Geometry: final body of the model. Coordinates: model frame, mm. A direction names the side the tool comes from. Coordinates: 2 decimals unless noted, no trailing zeros. Order: outer loops, then holes, each group sorted by start corner. A loop starts at its lowest first (then second) coordinate and runs counter-clockwise, first axis right, second up. Notation, with made-up numbers: M 41,88.5 L 87,88.5 A20 ccw 87,100.5 Z; hole C 82.25,89 d5. An arc over 180 degrees is marked long. Write item = value, one per line. Start each with the question number.
```python
from build123d import *

# Parameters (mm, degrees)
BOSS_EXTRUDE1_DEPTH    = 10
LPATTERN1_COUNT        = 2
LPATTERN1_PITCH        = 80
SKETCH2_W              = 69.30058394
SKETCH2_H              = 90
BOSS_EXTRUDE2_DEPTH    = 7
SKETCH3_R              = 2.5
CUT_EXTRUDE1_DEPTH     = 10
BOSS_EXTRUDE3_DEPTH    = 77
CUT_EXTRUDE2_START     = -2.5
CUT_EXTRUDE2_OUTLINE_W = 20.397762745
CUT_EXTRUDE2_OUTLINE_H = 50
CUT_EXTRUDE2_OUTLINE_R = 2.05
CUT_EXTRUDE2_DEPTH     = 2.5


# Read off the part's stored shape, not the designer's step: Cut-Extrude2
with BuildPart() as part:
    # Sketch1 → Boss-Extrude1 (new body)
    with BuildSketch(Plane.XY):
        Polygon((0, 0), (11.349310372, 59.718827606), (30.34970803, 100), (99.65029197, 100), (118.650689628, 59.718827606), (130, 0), (120, 0), (109.631710362, 54.556803995), (91.49827561, 93), (38.50172439, 93), (20.368289638, 54.556803995), (10, 0), align=None)
    extrude(amount=BOSS_EXTRUDE1_DEPTH)


with BuildPart() as lpattern1_1:
    # LPattern1: pattern copy
    add(part.part.moved(Location(Vector(0, 0, -1) * (1 * LPATTERN1_PITCH))))


with BuildPart() as part_1:
    add(part.part)

    add(lpattern1_1.part)  # Boss-Extrude2 merges LPattern1_1
    # Sketch2 → Boss-Extrude2 (add)
    with BuildSketch(Plane(origin=(0, 100, 0), x_dir=(1, 0, 0), z_dir=(0, 1, 0))):
        with Locations((65, 35)):
            Rectangle(SKETCH2_W, SKETCH2_H)
    extrude(amount=-BOSS_EXTRUDE2_DEPTH)

    # Sketch3 → Cut-Extrude1 (cut)
    with BuildSketch(Plane.XZ.offset(-93)):
        with Locations(Location((65, -35, 0), (0, 0, 270))):
            Circle(SKETCH3_R)
    extrude(amount=-CUT_EXTRUDE1_DEPTH, mode=Mode.SUBTRACT)

    # Sketch4 → Boss-Extrude3 (add)
    with BuildSketch(Plane.XY.offset(-70)):
        Polygon((130, 0), (129.524885584, 2.5), (119.524885584, 2.5), (120, 0), align=None)
        Polygon((0, 0), (10, 0), (10.475114416, 2.5), (0.475114416, 2.5), align=None)
    extrude(amount=BOSS_EXTRUDE3_DEPTH)

    # Cut-Extrude2 outline → Cut-Extrude2 (cut)
    with BuildSketch(Plane(origin=(0, 2.5, 0), x_dir=(1, 0, 0), z_dir=(0, 1, 0)).offset(CUT_EXTRUDE2_START)):
        with Locations((129.723766957, 35)):
            Rectangle(CUT_EXTRUDE2_OUTLINE_W, CUT_EXTRUDE2_OUTLINE_H)
        with Locations((0.276233043, 35)):
            Rectangle(CUT_EXTRUDE2_OUTLINE_W, CUT_EXTRUDE2_OUTLINE_H)
        with Locations((125, 65)):
            Circle(CUT_EXTRUDE2_OUTLINE_R)
        with Locations((125, 5)):
            Circle(CUT_EXTRUDE2_OUTLINE_R)
        with Locations((5, 5)):
            Circle(CUT_EXTRUDE2_OUTLINE_R)
        with Locations((5, 65)):
            Circle(CUT_EXTRUDE2_OUTLINE_R)
    extrude(amount=CUT_EXTRUDE2_DEPTH, mode=Mode.SUBTRACT)


solid = part_1.part
```
Item 1: Material intervals for probe 1 along Z at (x, y) = (125, 2); probe 2 along Z at (x, y) = (21, 69.5); probe 3 along Y at (x, z) = (78.5, -28.5), sorted ascending. Write a range as [from, to].
Item 2: Reachability of faces 1 (the flat face through (109.02, 80.14, 4.93)), 2 (the flat face through (100.69, 73.51, 4.93)), 3 (the flat face through (73, 93, -36)), 4 (the flat face through (8, 2.5, -65)) from +Z, -Z, +X, -X, +Y, -Y: full face, straight path, thin tool, end or side. Return the list, or none.
Item 3: Section query D-D on y = 38.5. Output: boundary loops of the cut face in (x, z).
Item 4: Draft query along Z for faces 5 (the flat face through (115, 51, 0)), 6 (the flat face through (100.69, 73.51, -75.07)). Return one class per face: pulls with the +Z half, pulls with the -Z half, needs draft (parallel to the pull), parting line crosses it, or undercut.
Item 5: First-contact query: pin 1 (7.5 mm diameter, centred on y = 98, z = -36, fed in from -X); pin 2 (8 mm diameter, centred on x = 99.5, z = -29, fed in from -Y); pin 3 (5.5 mm diameter, centred on y = 95.5, z = -51.5, fed in from +X). Flat tips, straight axial feed; report the tip coordinate or a pass-through.
Item 6: Section query A-A on z = -35. Output: boundary loops of the cut face in (x, y).
Item 7: Section query C-C on z = -65. Output: boundary loops of the cut face in (x, y), and give its area (3 significant figures).
Item 8: Section query B-B on x = 15. Output: boundary loops of the cut face in (y, z), and give its area (3 significant figures).
Ans:
q1.probe_1 = [-80, -67.05], [-62.95, -60], [-10, -7.05], [-2.95, 10]
q1.probe_2 = [-80, -70], [0, 10]
q1.probe_3 = [93, 100]
q2.face_1 = +Z, -Z, +X, +Y
q2.face_2 = +Z, -Z, -Y
q2.face_3 = -Y
q2.face_4 = +X, -X, +Y
q3.outline = M 7.32,-80 L 17.32,-80 L 17.32,-70 L 7.32,-70 Z; M 7.32,0 L 17.32,0 L 17.32,10 L 7.32,10 Z; M 112.68,-80 L 122.68,-80 L 122.68,-70 L 112.68,-70 Z; M 112.68,0 L 122.68,0 L 122.68,10 L 112.68,10 Z
q4.face_5 = undercut
q4.face_6 = needs draft
q5.pin_1 = 30.35
q5.pin_2 = 93
q5.pin_3 = 99.65
q6.outline = M 30.35,93 L 62.5,93 L 62.5,100 L 30.35,100 Z; M 67.5,93 L 99.65,93 L 99.65,100 L 67.5,100 Z
q7.outline = M 0,0 L 2.95,0 L 2.95,2.5 L 0.48,2.5 Z; M 7.05,0 L 10,0 L 10.48,2.5 L 7.05,2.5 Z; M 30.35,93 L 99.65,93 L 99.65,100 L 30.35,100 Z; M 119.52,2.5 L 120,0 L 122.95,0 L 122.95,2.5 Z; M 127.05,0 L 130,0 L 129.52,2.5 L 127.05,2.5 Z
q7.area = 515 mm^2
q8.outline = M 26.31,-80 L 67.46,-80 L 67.46,-70 L 26.31,-70 Z; M 26.31,0 L 67.46,0 L 67.46,10 L 26.31,10 Z
q8.area = 823 mm^2
